from build123d import *

# Parameters (mm, degrees)
SKETCH_2_R          = 2.25
CUT_EXTRUDE_1_DEPTH = 41.509258201
SKETCH_3_R          = 3.75
CUT_EXTRUDE_2_DEPTH = 4.1
CHAMFER_1_SIZE      = 0.5


with BuildPart() as part:
    # Эскиз1 → Повернуть1 (revolve)
    with BuildSketch(Plane.XY, mode=Mode.PRIVATE) as revolve_1_sk:
        Polygon((-5, 0), (-20, 0), (-20, 6), (-9.5, 6), (-9.5, 29), (-5, 29), align=None)
    revolve(revolve_1_sk.sketch.rotate(Axis((0, 0, 0), (0, 1, 0)), 270), axis=Axis((0, 0, 0), (0, 1, 0)))

    # Эскиз2 → Вырез-Вытянуть1 (cut, through all)
    with BuildSketch(Plane.XZ):
        with Locations(Location((0, 14.5, 0), (0, 0, 270))):
            Circle(SKETCH_2_R)
        with Locations(Location((14.5, 0, 0), (0, 0, 270))):
            Circle(SKETCH_2_R)
        with Locations(Location((0, -14.5, 0), (0, 0, 270))):
            Circle(SKETCH_2_R)
        with Locations(Location((-14.5, 0, 0), (0, 0, 270))):
            Circle(SKETCH_2_R)
    extrude(amount=-CUT_EXTRUDE_1_DEPTH, mode=Mode.SUBTRACT)

    # Эскиз3 → Вырез-Вытянуть2 (cut)
    with BuildSketch(Plane.XZ):
        with Locations(Location((0, 14.5, 0), (0, 0, 270))):
            Circle(SKETCH_3_R)
        with Locations(Location((14.5, 0, 0), (0, 0, 270))):
            Circle(SKETCH_3_R)
        with Locations(Location((0, -14.5, 0), (0, 0, 270))):
            Circle(SKETCH_3_R)
        with Locations(Location((-14.5, 0, 0), (0, 0, 270))):
            Circle(SKETCH_3_R)
    extrude(amount=-CUT_EXTRUDE_2_DEPTH, mode=Mode.SUBTRACT)

    # Фаска1
    chamfer_1_edges = [part.edges().sort_by_distance(p)[0] for p in [
        (0, 29, 9.5),
        (0, 6, 20),
        (0, 0, 20),
    ]]
    chamfer(chamfer_1_edges, length=CHAMFER_1_SIZE)


solid = part.part
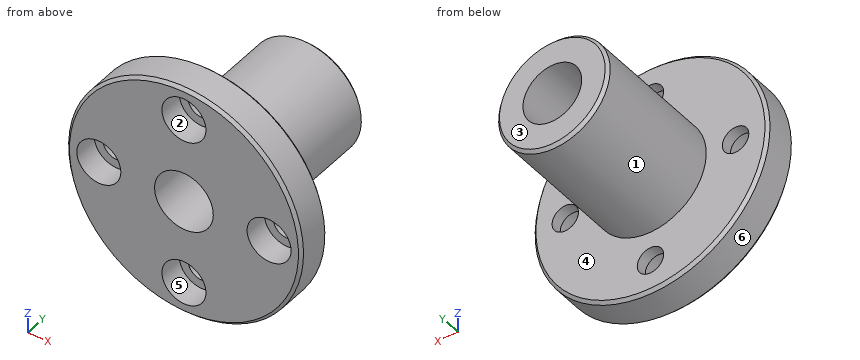
Verification items for the finished model (mm, model axes). Face numbers are marked on the shaded views. A direction names the side the tool comes from. Round coordinates to 2 decimals unless told otherwise and drop trailing zeros. Order: outer loops, then holes, each group sorted by start corner. A loop starts at its lowest first (then second) coordinate and runs counter-clockwise, first axis right, second up. Notation, with made-up numbers: (77.5, 0) -> (92.5, 0) arc R25 ccw to (92.5, 31) -> close; hole circle Ø3 at (71, 84). An arc over 180 degrees is marked (long way). Put each result on its own line as item: value.
1) Set-up check for the marked faces 4, 5 and 6: record each of +Z, -Z, +X, -X, +Y, -Y from which the full face is reachable in a straight line by a thin tool's end or side.
Final values:
face 4: +Y
face 5: -Y
face 6: +Y, -Y
2) Depth check by flat-ended pin: pin 1 (7 mm diameter, centred on x = -14.5, z = 0, fed in from +Y); pin 2 (6 mm diameter, centred on x = 6.5, y = 9.5, fed in from +Z); pin 3 (10 mm diameter, centred on y = 19.5, z = -5, fed in from +X). Enter the tip coordinate at first touch or a pass-through.
Final values:
pin 1: stops at y = 6
pin 2: stops at z = 8.83
pin 3: stops at x = 9.5
3) Material ranges on line 1 (X direction, y = 4.5, z = 0); line 2 (Y direction, x = -2, z = 12.5); line 3 (Y direction, x = -6.5, z = -8.5), recorded low to high.
Final values:
line 1: x = -20 to -16.75, -12.25 to -5, 5 to 12.25, 16.75 to 20
line 2: y = 4.1 to 6
line 3: y = 0 to 6
4) Mould release check, pull along X, two halves, no side actions. Record for the marked faces 1, 2 and 3: +X half, -X half, draft (parallel to the pull), parting line (faces both ways), or undercut.
Final values:
face 1: parting line
face 2: undercut
face 3: draft
5) Section check C-C (y = 25.25). Record the cut outline in (x, z).
Final values:
outline: circle Ø19 at (0, 0); hole circle Ø10 at (0, 0)
6) Section check A-A (x = 0). Give the number of separate pieces and of enclosed holes in the cut face, then the cut area to 3 significant figures.
Final values:
separate pieces: 4
enclosed holes: 0
area: 308 mm^2
